```python
from build123d import *

# Parameters (mm, degrees)
SKETCH1_R           = 12.7
BOSS_EXTRUDE1_DEPTH = 25.4
SKETCH2_R           = 15.24
BOSS_EXTRUDE2_DEPTH = 3.1496
FILLET1_R           = 3.81
SKETCH5_W           = 6.35
SKETCH5_H           = 6.35
CUT_EXTRUDE2_DEPTH  = 12.7


with BuildPart() as part:
    # Sketch1 → Boss-Extrude1 (new body)
    with BuildSketch(Plane(origin=(0, 0, 0), x_dir=(0, 0, -1), z_dir=(1, 0, 0))):
        Circle(SKETCH1_R)
    extrude(amount=BOSS_EXTRUDE1_DEPTH)

    # Sketch2 → Boss-Extrude2 (add)
    with BuildSketch(Plane(origin=(25.4, 0, 0), x_dir=(0, 0, -1), z_dir=(1, 0, 0))):
        Circle(SKETCH2_R)
    extrude(amount=BOSS_EXTRUDE2_DEPTH)

    # Fillet1
    # the kernel refuses this fillet: 3.81 mm, written as the material it takes off along each edge
    with BuildSketch(Plane(origin=(28.5496, 0, 0), x_dir=(0, 0, -1), z_dir=(0, -1, 0))) as fillet1_piece_1:
        with BuildLine():
            CenterArc((11.487671144, -3.81), FILLET1_R, 9.98168298, 80.01831702)
            Line((11.487671144, 0), (11.487671144, 0.0762))
            Line((11.487671144, 0.0762), (15.24, 0.0762))
            Line((15.24, 0.0762), (15.3162, 0))
            ThreePointArc((15.3162, 0), (15.3162, -1.5748), (15.315046577, -3.136392))
            Line((15.315046577, -3.136392), (15.24, -3.1496))
        make_face()
    revolve(axis=Axis((28.5496, 0, 0), (1, 0, 0)), mode=Mode.SUBTRACT)

    # Sketch5 → Cut-Extrude2 (cut)
    with BuildSketch(Plane(origin=(28.5496, 0, 0), x_dir=(0, 0, -1), z_dir=(1, 0, 0))):
        Rectangle(SKETCH5_W, SKETCH5_H)
    extrude(amount=-CUT_EXTRUDE2_DEPTH, mode=Mode.SUBTRACT)


solid = part.part
```
For this review, take the finished solid that the model builds, in its own axes (mm). A direction names the side the tool comes from. Give positions to 0.01 mm unless a question says otherwise; leave off trailing zeros. Write each loop counter-clockwise with the first axis right and the second up, starting at its lowest first coordinate (ties: lowest second). Pieces come first, ordered by that corner, then holes.
Item 1: Insertion check: P1, Ø1, axis at y = 9, z = 3, coming from the -X side; P2, Ø4, axis at x = 6, y = -4, coming from the +Z side; P3, Ø7, axis at x = 20, y = -1, coming from the +Z side; P4, Ø1.9, axis at x = 23.5, z = 0, coming from the +Y side. Each pin has a flat end and moves straight along its axis. Give the tip position at first contact, or say it passes through.
Item 2: Take a section at A-A (y = 0). Give the boundary of the cut face in (x, z) (3 decimals).
Item 3: The part is to be moulded in two halves that separate along Z. For faces 4 (the face through (12.52, -12.4, 2.75)), 5 (the face through (0, 0, 0)), 6 (the face through (22, 0, -3.175)), say which applies: +Z half, -Z half, draft (parallel to the pull), parting line (faces both ways), or undercut.
Item 4: Machinability: for faces 1 (the face through (28.55, -5, 0)), 2 (the face through (25.4, 12.5, 3.5)), 3 (the face through (15.85, 0, 0)), which of the approach directions +Z, -Z, +X, -X, +Y, -Y give a long, thin tool a straight path to every point of the face, cutting with its end or side? Answer none if there is none.
Item 5: Take a section at C-C (x = 5). Give the boundary of the cut face in (y, z), and give its area (3 significant figures).
Item 6: Wall thickness on probe 1 along X at (y, z) = (5, -10.5); probe 2 along X at (y, z) = (13, -6.5); probe 3 along Z at (x, y) = (3, -2): over which ranges is each line inside the solid? List them lowest first.
Established:
1. P1: stops at x = 0
1. P2: stops at z = 12.54
1. P3: stops at z = 12.7
1. P4: stops at y = 12.7
2. outline: (0, -12.7) - (25.4, -12.7) - (25.4, -15.24) arc R3.81 ccw to (28.55, -11.488) - (28.55, -3.175) - (15.85, -3.175) - (15.85, 3.175) - (28.55, 3.175) - (28.55, 11.488) arc R3.81 ccw to (25.4, 15.24) - (25.4, 12.7) - (0, 12.7) - close
3. face 4: parting line
3. face 5: draft
3. face 6: undercut
4. face 1: +Z, -Z, +X, +Y, -Y
4. face 2: -X
4. face 3: +X
5. outline: circle Ø25.4 at (0, 0)
5. area: 507 mm2
6. probe 1: x = 0 to 28.55
6. probe 2: x = 25.4 to 27.03
6. probe 3: z = -12.54 to 12.54
